from build123d import *

# Parameters (mm, degrees)
F0_R     = 9
F1_DEPTH = 4
F3_W     = 3
F3_H     = 3
F4_DEPTH = 2
F2_R     = 9
F2_R_2   = 8
F5_DEPTH = 1
F7_DEPTH = 1


# Not quite as in the source:
# - a feature names something its author has since deleted; it is built from what else it names


with BuildPart() as f1:
    # F0 (on Top) → F1 (new body)
    with BuildSketch(Plane.XY):
        with Locations((-31.3306450844, 19.7580661625)):
            Circle(F0_R)
    extrude(amount=F1_DEPTH)

    # F3 (on face) → F4 (cut)
    with BuildSketch(Plane(origin=(0, 0, 0), x_dir=(1, 0, 0), z_dir=(0, 0, -1))):
        with BuildLine():
            ThreePointArc((-32.8306450844, -28.6321858371), (-32.0832814269, -28.7265408676), (-31.3306450844, -28.7580661625))
            ThreePointArc((-31.3306450844, -28.7580661625), (-30.5780087419, -28.7265408676), (-29.8306450844, -28.6321858371))
            Line((-29.8306450844, -28.6321858371), (-29.8306450844, -21.2580661625))
            Line((-29.8306450844, -21.2580661625), (-32.8306450844, -21.2580661625))
            Line((-32.8306450844, -21.2580661625), (-32.8306450844, -28.6321858371))
        make_face()
        with BuildLine():
            ThreePointArc((-40.204764759, -18.2580661625), (-40.2991197895, -19.0054298199), (-40.3306450844, -19.7580661625))
            ThreePointArc((-40.3306450844, -19.7580661625), (-40.2991197895, -20.510702505), (-40.204764759, -21.2580661625))
            Line((-40.204764759, -21.2580661625), (-32.8306450844, -21.2580661625))
            Line((-32.8306450844, -21.2580661625), (-32.8306450844, -18.2580661625))
            Line((-32.8306450844, -18.2580661625), (-40.204764759, -18.2580661625))
        make_face()
        with Locations((-31.3306450844, -19.7580661625)):
            Rectangle(F3_W, F3_H)
        with BuildLine():
            Line((-29.8306450844, -18.2580661625), (-29.8306450844, -21.2580661625))
            Line((-29.8306450844, -21.2580661625), (-22.4565254097, -21.2580661625))
            ThreePointArc((-22.4565254097, -21.2580661625), (-22.3621703793, -20.510702505), (-22.3306450844, -19.7580661625))
            ThreePointArc((-22.3306450844, -19.7580661625), (-22.3621703793, -19.0054298199), (-22.4565254097, -18.2580661625))
            Line((-22.4565254097, -18.2580661625), (-29.8306450844, -18.2580661625))
        make_face()
        with BuildLine():
            Line((-32.8306450844, -10.8839464878), (-32.8306450844, -18.2580661625))
            Line((-32.8306450844, -18.2580661625), (-29.8306450844, -18.2580661625))
            Line((-29.8306450844, -18.2580661625), (-29.8306450844, -10.8839464878))
            ThreePointArc((-29.8306450844, -10.8839464878), (-30.5780087419, -10.7895914574), (-31.3306450844, -10.7580661625))
            ThreePointArc((-31.3306450844, -10.7580661625), (-32.0832814269, -10.7895914574), (-32.8306450844, -10.8839464878))
        make_face()
    extrude(amount=-F4_DEPTH, mode=Mode.SUBTRACT)

    # F2 (on face) → F5 (join)
    with BuildSketch(Plane.XY.offset(4)):
        with Locations((-31.3306450844, 19.7580661625)):
            Circle(F2_R)
        with Locations((-31.3306450844, 19.7580661625)):
            Circle(F2_R_2, mode=Mode.SUBTRACT)
    extrude(amount=F5_DEPTH)

    # F6 (on face) → F7 (join)
    with BuildSketch(Plane.XY.offset(4)):
        Polygon((-31.8826989997, 17.620101061), (-31.6466835645, 17.6265811855), (-31.7066879875, 16.579484876), (-31.6994015259, 15.6946153355), (-31.6409921199, 14.9638444516), (-31.5461033208, 14.3823088935), (-31.5023139233, 14.1560195308), (-31.4098559066, 14.0027283885), (-31.2557513645, 13.9021557962), (-31.0951431551, 14.0935678455), (-30.9597079636, 15.2290645897), (-30.9069900022, 17.6882277109), (-29.3254158456, 17.7312048856), (-26.5207167102, 17.7758241628), (-26.2806401616, 17.8001378726), (-26.131438384, 17.902336676), (-26.1387366169, 18.0799662479), (-26.2968846155, 18.3046282224), (-26.7843359457, 18.5990530635), (-27.2012180722, 18.7815383146), (-27.5588903414, 18.842378503), (-27.8670641117, 18.7685604085), (-29.2313039551, 18.5276657515), (-30.9069900022, 18.2916503163), (-30.9264421472, 18.7580132848), (-30.9199620226, 19.2844101047), (-29.6028075528, 19.3979623688), (-29.6133429052, 19.3346972837), (-29.5768517406, 19.3103600312), (-29.5127567758, 19.1319241223), (-29.336775192, 19.0962275234), (-29.1826294501, 19.1457083654), (-29.0253054456, 19.3103600312), (-28.7941751179, 19.7483540621), (-28.4575735534, 20.6534526562), (-28.1363924487, 21.2779812803), (-27.6789580441, 21.7857381779), (-27.5499441205, 22.0039200278), (-27.6172762047, 22.239935463), (-27.9798335815, 22.5019067104), (-28.5711081605, 22.8758234335), (-28.9742178152, 22.9277350579), (-29.6644305355, 22.8142004508), (-30.9329399287, 22.6389840043), (-30.8940120961, 23.59281596), (-29.4016352941, 23.8685596792), (-28.9044726056, 23.9918645013), (-28.6586869554, 24.0956877501), (-28.5857046263, 24.1807945629), (-28.5970639727, 24.3098084866), (-28.7698084371, 24.4362915714), (-29.0609726161, 24.562833513), (-29.4551949066, 24.5750168534), (-29.829876767, 24.5109218886), (-30.3684157276, 24.3390014182), (-30.88103419, 24.1962150228), (-30.890769091, 24.1840316823), (-30.8680562839, 24.222170835), (-30.8137197628, 24.6561214094), (-30.6182036345, 25.065705303), (-30.6417463214, 25.2798260395), (-30.8064097585, 25.4907096565), (-31.2273471128, 25.7194268588), (-31.7245451154, 25.8929953172), (-31.9767755761, 25.897821568), (-32.162527375, 25.7696904951), (-32.222531798, 25.6293760818), (-32.1138587557, 25.4907096565), (-31.8267439188, 25.1127318199), (-31.6856113971, 24.6731310006), (-31.6985893032, 24.3657223677), (-31.672633491, 24.021057433), (-33.2688158848, 23.8198851742), (-33.5632230689, 23.7177099135), (-33.4083239611, 23.5311341206), (-32.8202865015, 23.3291967246), (-32.0003006059, 23.4046510358), (-31.672633491, 23.4435553257), (-31.6904729619, 22.9942431481), (-31.672633491, 22.5124420627), (-32.0514000076, 22.4338094888), (-32.363658434, 22.3891960973), (-33.186075112, 22.2423485884), (-33.8495492258, 22.1523566681), (-34.4399939251, 22.3405215924), (-34.6022089228, 22.288609968), (-34.648440874, 22.167777128), (-34.5535461892, 22.0614818971), (-34.1845028022, 21.2650328026), (-33.8235934136, 19.9267487714), (-33.6346044953, 19.2146413523), (-33.2071693594, 18.7815383146), (-33.1990530181, 18.7555883881), (-33.1682415268, 18.7685604085), (-33.0336126723, 18.7896605415), (-32.954109019, 19.0086487285), (-32.8770773478, 18.9867422584), (-32.7659499804, 19.0216266346), (-32.2825597636, 19.1213711129), (-31.6369427778, 19.1968077671), (-31.6612800303, 18.6485280198), (-31.6466835645, 18.1781157092), (-33.8868408417, 17.9031488987), (-36.2730075081, 17.6622718987), (-36.4798311888, 17.5673595569), (-36.3638475537, 17.360560596), (-35.8309782607, 17.0328699384), (-35.2802618454, 17.0328699384), (-34.2810337038, 17.2680790366), (-33.4042569619, 17.4465208312), (-32.654822613, 17.560885318), (-32.0392343242, 17.6006253733), align=None)
        Polygon((-31.6758764961, 21.5699694534), (-31.6466835645, 21.0817529858), (-32.1901017469, 20.936553465), (-32.6523977163, 20.8546249149), (-32.7691870998, 20.7483885407), (-32.6167011174, 20.6177854857), (-32.4601716785, 20.5391529118), (-32.2273933628, 20.5529253835), (-31.6466835645, 20.6307928201), (-31.6653293724, 20.1173856777), (-31.6369427778, 19.6380271461), (-32.3620398743, 19.524474882), (-32.9930603943, 19.4368960871), (-33.1552636207, 20.0500535935), (-33.3628983469, 21.1125350488), (-33.4472400224, 21.6591962363), (-32.6832268646, 21.8351778202), (-31.6596614706, 22.0387632043), align=None, mode=Mode.SUBTRACT)
        Polygon((-30.9329399287, 19.7743098743), (-30.9329399287, 20.718371615), (-30.0180416913, 20.8449135566), (-29.8485343463, 20.8919400735), (-29.829876767, 21.0460269586), (-30.0180416913, 21.1847522406), (-30.2775998133, 21.3088222), (-30.5720011117, 21.318592415), (-30.9329399287, 21.2569105756), (-30.9329399287, 22.1523566681), (-30.2143288425, 22.2545319288), (-29.6530711891, 22.3080915413), (-29.2556706359, 22.3120937981), (-29.0253054456, 22.2626541558), (-28.9636824629, 22.070428118), (-28.9864011556, 21.7370636729), (-29.1802163247, 21.0022375611), (-29.328652965, 20.4287965674), (-29.4438355602, 20.0159755543), (-29.537888594, 19.7613025399), (-30.1016182294, 19.8886684755), align=None, mode=Mode.SUBTRACT)
    extrude(amount=F7_DEPTH)


solid = f1.part
The listing builds one solid part. Answer for the finished solid, in the listing's coordinates (mm). A direction names the side the tool comes from. Coordinates: 2 decimals unless noted, no trailing zeros. Write each loop counter-clockwise with the first axis right and the second up, starting at its lowest first coordinate (ties: lowest second). Pieces come first, ordered by that corner, then holes. Notation, with made-up numbers: (39.25, 20.25) - (73.25, 20.25) arc R20 cw to (73.25, 34.25) - close; hole circle Ø1 at (69.5, 33.5). An arc over 180 degrees is marked (long way). Return JSON: item names as keys, results as strings.
1. Consider line 1 along Z through (x, y) = (-29.75, 18.75); line 2 along Z through (x, y) = (-28.75, 26.75); line 3 along Y through (x, z) = (-24.25, 0.5). Determine where each line is inside the solid, lowest interval first.
Final values:
{"line 1": "2 to 4", "line 2": "0 to 4", "line 3": "14.2 to 18.26, 21.26 to 25.31"}
2. The part is cut by section B-B on x = -38.5. Determine the outline of the cut face in (y, z), then the cut area to 3 significant figures.
Final values:
{"outline": "(14.32, 0) - (18.26, 0) - (18.26, 2) - (21.26, 2) - (21.26, 0) - (25.2, 0) - (25.2, 5) - (23.31, 5) - (23.31, 4) - (16.21, 4) - (16.21, 5) - (14.32, 5) - close", "area": "41.3 mm^2"}
3. Each of these flat-tipped pins is pushed along its axis until it touches: pin 1 Ø1 at (y, z) = (22, 4.5) entering from +X; pin 2 Ø2 at (y, z) = (25, 0.5) entering from +X; pin 3 Ø0.6 at (x, z) = (-24.5, 0.5) entering from +Y; pin 4 Ø1.5 at (x, y) = (-24.5, 21) entering from -Z. Where does it stop, or does it pass through?
Final values:
{"pin 1": "x = -22.5", "pin 2": "x = -23.39", "pin 3": "y = 25.95", "pin 4": "z = 0"}
4. Which of the six approach directions +Z, -Z, +X, -X, +Y, -Y give full straight-line access (tool end or side, diameter ignored) to faces 1 (the face through (-39, 16, 5)), 2 (the face through (-29.831, 15, 1)), 3 (the face through (-32.769, 22.317, 4.493))?
Final values:
{"face 1": "+Z, +X, -X, +Y, -Y", "face 2": "-Z, +Y, -Y", "face 3": "+Z"}
5. For a pull along X with two mould halves and no side action, classify faces 4 (the face through (-26, 21.258, 1)), 5 (the face through (-27.178, 11.774, 2.465)), 6 (the face through (-30.914, 23.109, 4.493)) as +X half, -X half, draft (parallel to the pull), parting line (faces both ways), or undercut.
Final values:
{"face 4": "draft", "face 5": "parting line", "face 6": "undercut"}
6. The part is cut by section A-A on y = 12. Determine the outline of the cut face in (x, z), then the cut area to 3 significant figures.
Final values:
{"outline": "(-35.89, 0) - (-32.83, 0) - (-32.83, 2) - (-29.83, 2) - (-29.83, 0) - (-26.77, 0) - (-26.77, 5) - (-29.38, 5) - (-29.38, 4) - (-33.28, 4) - (-33.28, 5) - (-35.89, 5) - close", "area": "35.7 mm^2"}
7. The part is cut by section D-D on z = 2.85. Determine the outline of the cut face in (x, y), then the cut area to 3 significant figures.
Final values:
{"outline": "circle Ø18 at (-31.33, 19.76)", "area": "254 mm^2"}
8. The part is cut by section C-C on y = 16. Determine the outline of the cut face in (x, z), then the cut area to 3 significant figures.
Final values:
{"outline": "(-39.51, 0) - (-32.83, 0) - (-32.83, 2) - (-29.83, 2) - (-29.83, 0) - (-23.15, 0) - (-23.15, 5) - (-24.27, 5) - (-24.27, 4) - (-30.94, 4) - (-30.94, 5) - (-31.7, 5) - (-31.7, 4) - (-38.39, 4) - (-38.39, 5) - (-39.51, 5) - close", "area": "62.4 mm^2"}
